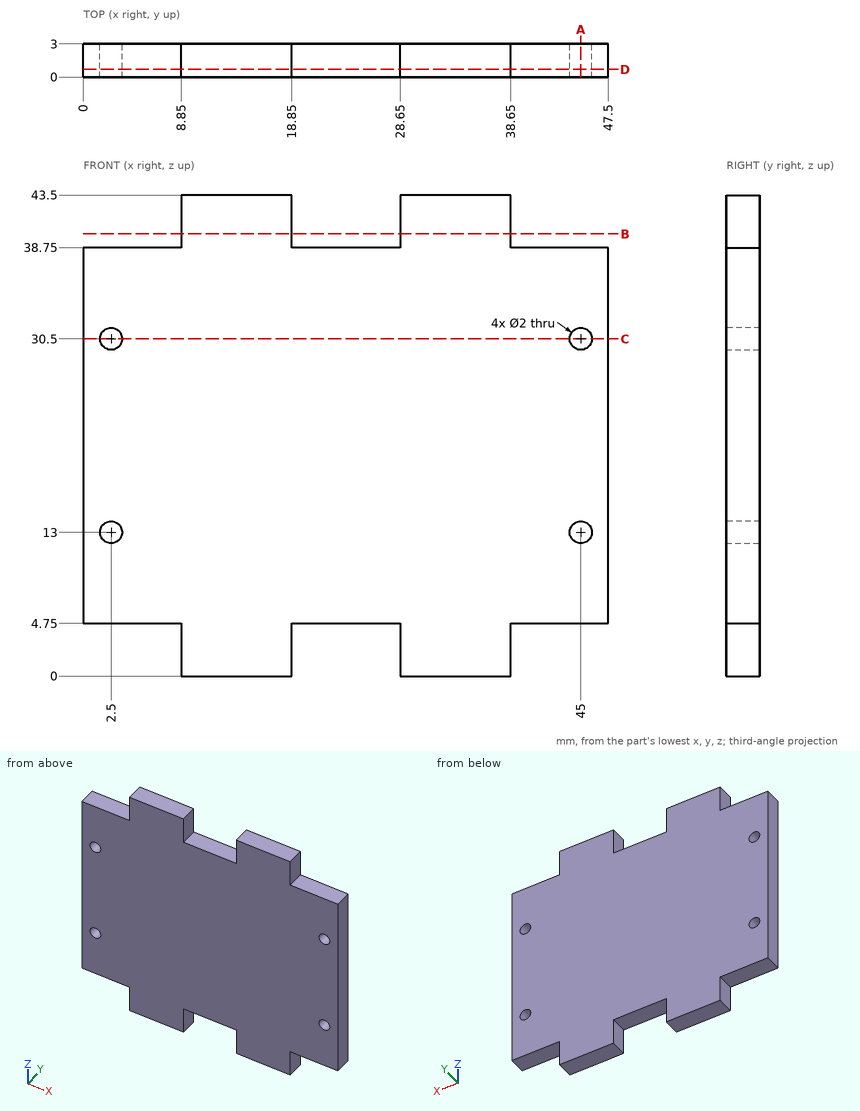
Here's the drawing with two shaded views (mm, measured from the low corner). I have some questions. Round coordinates to 2 decimals unless told otherwise and drop trailing zeros. Order: outer loops, then holes, each group sorted by start corner. A loop starts at its lowest first (then second) coordinate and runs counter-clockwise, first axis right, second up. Notation, with made-up numbers: (15.5, -1) -> (71.5, -1) arc R21 ccw to (71.5, 4) -> close; hole circle Ø1 at (74.5, -37). An arc over 180 degrees is marked (long way). Return JSON: item names as keys, results as strings.
Q1. I need wall thicknesses on line 1 along X through (y, z) = (1, 30.5); line 2 along Z through (x, y) = (45, 0.6); line 3 along X through (y, z) = (1.55, 4). Which ranges of each line are inside material? Lowest first, please. Write a range as from..to.
Filled sheet:
{"line 1": "x = 0..1.5, 3.5..44, 46..47.5", "line 2": "z = 4.75..12, 14..29.5, 31.5..38.75", "line 3": "x = 8.85..18.85, 28.65..38.65"}
Q2. If we section it at B-B on z = 40: List the corners of the cut face in (x, y) for me, plus the area to 3 significant figures.
Filled sheet:
{"outline": "(8.85, 0) -> (18.85, 0) -> (18.85, 3) -> (8.85, 3) -> close; (28.65, 0) -> (38.65, 0) -> (38.65, 3) -> (28.65, 3) -> close", "area": "60.0 mm^2"}
Q3. For pin 1 Ø1.5 at (y, z) = (1, 3.5) entering from +X; pin 2 Ø1.5 at (y, z) = (1.5, 41) entering from -X, each with a flat end and sliding along its axis, tell me the tip position at first contact or that it passes through.
Filled sheet:
{"pin 1": "stops at x = 38.65", "pin 2": "stops at x = 8.85"}
Q4. If we section it at D-D on y = 0.7: List the corners of the cut face in (x, z) for me, plus the area to 3 significant figures.
Filled sheet:
{"outline": "(0, 4.75) -> (8.85, 4.75) -> (8.85, 0) -> (18.85, 0) -> (18.85, 4.75) -> (28.65, 4.75) -> (28.65, 0) -> (38.65, 0) -> (38.65, 4.75) -> (47.5, 4.75) -> (47.5, 38.75) -> (38.65, 38.75) -> (38.65, 43.5) -> (28.65, 43.5) -> (28.65, 38.75) -> (18.85, 38.75) -> (18.85, 43.5) -> (8.85, 43.5) -> (8.85, 38.75) -> (0, 38.75) -> close; hole circle Ø2 at (2.5, 13); hole circle Ø2 at (2.5, 30.5); hole circle Ø2 at (45, 13); hole circle Ø2 at (45, 30.5)", "area": "1,790 mm^2"}
Q5. If we section it at C-C on z = 30.5: List the corners of the cut face in (x, y) for me.
Filled sheet:
{"outline": "(0, 0) -> (1.5, 0) -> (1.5, 3) -> (0, 3) -> close; (3.5, 0) -> (44, 0) -> (44, 3) -> (3.5, 3) -> close; (46, 0) -> (47.5, 0) -> (47.5, 3) -> (46, 3) -> close"}
Q6. If we section it at A-A on x = 45: List the corners of the cut face in (y, z) for me.
Filled sheet:
{"outline": "(0, 4.75) -> (3, 4.75) -> (3, 12) -> (0, 12) -> close; (0, 14) -> (3, 14) -> (3, 29.5) -> (0, 29.5) -> close; (0, 31.5) -> (3, 31.5) -> (3, 38.75) -> (0, 38.75) -> close"}
